Check sheet for the modelled part. Datum: model origin and axes. Units: mm. Coordinates: 2 decimals unless noted, no trailing zeros. Loops run counter-clockwise (first coordinate to the right, second up) from the corner with the lowest first, then second, coordinate; pieces in that order, holes last. Notation, with made-up numbers: M 87,-38.75 L 125,-38.75 A31 ccw 125,-1.75 Z; hole C 85.5,8 d3. An arc over 180 degrees is marked long. Return JSON: item names as keys, results as strings.
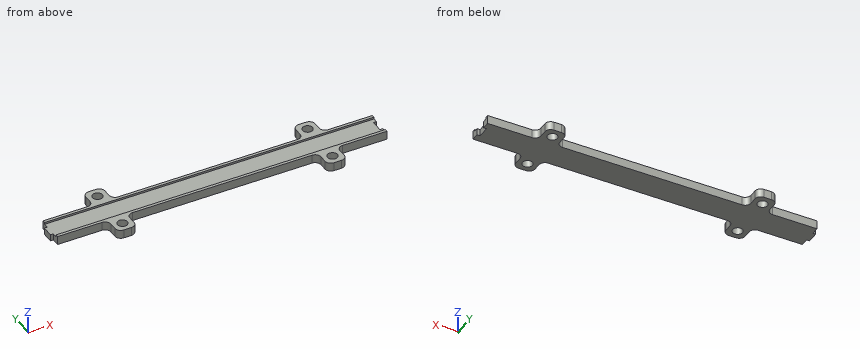
Autodesk Inventor part; units mm, degrees
ref_plane "YZ Plane" through (0, 0, 0) normal (1, 0, 0) x (0, 1, 0)
ref_plane "XZ Plane" through (0, 0, 0) normal (0, 1, 0) x (-1, 0, 0)
ref_plane "XY Plane" through (0, 0, 0) normal (0, 0, 1) x (1, 0, 0)
sketch "Skizze2" plane through (0, 0, 0) normal (0, 0, 1) x (1, 0, 0)
  line L0 (-86.25, 7) -> (86.25, 7)
  line L1 (86.25, 7) -> (86.25, -7)
  line L2 (86.25, -7) -> (-86.25, -7)
  line L3 (-86.25, -7) -> (-86.25, 7)
  line L4 (0, 9.8) -> (0, -9.8)
  line L5 (-120.75, 0) -> (120.75, 0)
  point P0 (0, 0)
  point P1 (-86.25, 0)
  point P2 (0, 7)
  dimension "d0" = 14
  dimension "d1" = 172.5
extrude "Extrusion1" add sketch "Skizze2" along normal blind 3.5
sketch "Skizze3" plane through (0, 0, 3.5) normal (0, 0, 1) x (1, 0, 0)
  line L0 (86.25, -7) -> (86.25, 7)
  line L1 (86.25, 7) -> (-86.25, 7)
  line L2 (-86.25, 7) -> (-86.25, -7)
  line L3 (-86.25, -7) -> (86.25, -7)
  line L4 (86.25, 7) -> (-86.25, 7)
  line L5 (-86.25, 7) -> (-86.25, 5.5)
  line L6 (-86.25, 5.5) -> (86.25, 5.5)
  line L7 (86.25, 5.5) -> (86.25, 7)
  line L8 (-86.25, 7) -> (-86.25, -7)
  line L9 (-86.25, -7) -> (86.25, -7)
  line L10 (86.25, -7) -> (86.25, -5.5)
  line L11 (86.25, -5.5) -> (-86.25, -5.5)
  line L12 (-86.25, -5.5) -> (-86.25, -7)
  point P0 (0, 0)
  dimension "d4" = 1.5
  dimension "d5" = 1.5
extrude "Extrusion2" add sketch "Skizze3" along normal blind 1 contours L3 L2 L11 L0 | L6 L2 L1 L0
sketch "Skizze4" plane through (0, 0, 0) normal (0, 0, -1) x (-1, 0, 0)
  line L0 (86.25, -7) -> (-86.25, -7)
  line L1 (155.9309, -7) -> (147.0048, -7)
  line L2 (60, -7) -> (50, -7)
  line L3 (50, -7) -> (50, -17)
  line L4 (50, -17) -> (60, -17)
  line L5 (60, -17) -> (60, -7)
  line L6 (50, 7) -> (60, 7)
  line L7 (60, 7) -> (60, 17)
  line L8 (60, 17) -> (50, 17)
  line L9 (50, 17) -> (50, 7)
  line L10 (86.25, -7) -> (-86.25, -7)
  line L11 (-86.25, 7) -> (86.25, 7)
  line L12 (86.25, 7) -> (86.25, -7)
  line L13 (-60, -9.0118) -> (-60, -17) construction
  line L14 (-60, -17) -> (-50, -17) construction
  line L15 (-50, -17) -> (-50, -7) construction
  line L16 (-86.25, -7) -> (-86.25, 7)
  point P0 (0, 0)
  point P1 (50, -7)
  point P2 (55, -17)
  point P3 (-55, -17)
  point P4 (55, -12)
  point P5 (55, 12)
  point P6 (60, -12)
  point P7 (60, 12)
  dimension "d8" = 10
  dimension "d9" = 10
  dimension "d30" = 110
  dimension "d31" = 10
  dimension "d32" = 24
  dimension "d33" = 55
extrude "Extrusion3" add sketch "Skizze4" against normal up to surface (4.5 mm away) contours L5 L4 L3 L0 | L6 L9 L8 L7
sketch "Skizze5" plane through (0, 0, 0) normal (0, 0, -1) x (-1, 0, 0)
  line L0 (50, -17) -> (60, -17)
  line L1 (50, -7) -> (50, -17)
  line L2 (50, 17) -> (50, 7)
  point P0 (0, 0)
  point P1 (55, -12)
  point P2 (55, 12)
  point P3 (55, -17)
  point P4 (50, -12)
  point P5 (50, 12)
  dimension "d13" = 24
hole "Bohrung1" at (-55, -12, 0) direction (0, 0, 1) diameter 5.2 end through all
fillet "Rundung1" radius 3 8 edges at (-60, -17, 2.25) (-50, -17, 2.25) (-50, -7, 2.25) (-60, -7, 2.25) (-50, 17, 2.25) (-60, 17, 2.25) (-50, 7, 2.25) (-60, 7, 2.25)
pattern_linear "Rechteckige Anordnung1" count 2 spacing 24 along (0, 1, 0) of "Bohrung1"
pattern_linear "Rechteckige Anordnung2" count 2 spacing 110 along (1, 0, 0) of "Rundung1", "Bohrung1", "Extrusion3", "Rechteckige Anordnung1"
sketch "Skizze7" plane through (0, 0, 3.5) normal (0, 0, 1) x (1, 0, 0)
  line L0 (-86.25, 5.5) -> (-86.25, -5.5)
  line L1 (-86.25, 3) -> (-87.75, 3)
  line L2 (-87.75, 3) -> (-87.75, -3)
  line L3 (-87.75, -3) -> (-86.25, -3)
  line L4 (-86.25, -3) -> (-86.25, 3)
  line L5 (86.25, -3.1) -> (84.65, -3.1)
  line L6 (84.65, -3.1) -> (84.65, 3.1)
  line L7 (84.65, 3.1) -> (86.25, 3.1)
  line L8 (86.25, 3.1) -> (86.25, -3.1)
  line L9 (86.25, -5.5) -> (86.25, 5.5)
  point P0 (0, 0)
  point P1 (-87.75, 0)
  point P2 (-86.25, 0)
  point P3 (-86.25, 0)
  point P4 (84.65, 0)
  point P5 (86.25, 0)
  point P6 (86.25, 0)
  dimension "d37" = 1.5
  dimension "d38" = 6
  dimension "d41" = 1.6
  dimension "d44" = 6.2
extrude "Extrusion5" add sketch "Skizze7" against normal up to surface (3.5 mm away) contours L0 L3 L2 L1
extrude "Extrusion6" cut sketch "Skizze7" against normal through all contours L5 L6 L7 L8
equation "\"d5\" = d4"
equation "\"d9\" = d8"
equation "\"d24\" = d13"
properties part number "LED_Strip_Halter" material "PA 6 schwarz"
1) Section check C-C on z = 2. Count the separate pieces of the cut face and the enclosed holes in it, then the cut area to 3 significant figures.
Answers:
{"separate pieces": "1", "enclosed holes": "4", "area": "2,730 mm²"}
2) Section check A-A on y = -12. Record the cut outline in (x, z).
Answers:
{"outline": "M -60,0 L -57.6,0 L -57.6,4.5 L -60,4.5 Z; M -52.4,0 L -50,0 L -50,4.5 L -52.4,4.5 Z; M 50,0 L 52.4,0 L 52.4,4.5 L 50,4.5 Z; M 57.6,0 L 60,0 L 60,4.5 L 57.6,4.5 Z"}
3) Section check B-B on x = -55. Record the cut outline in (y, z).
Answers:
{"outline": "M -17,0 L -14.6,0 L -14.6,4.5 L -17,4.5 Z; M -9.4,0 L 9.4,0 L 9.4,4.5 L 5.5,4.5 L 5.5,3.5 L -5.5,3.5 L -5.5,4.5 L -9.4,4.5 Z; M 14.6,0 L 17,0 L 17,4.5 L 14.6,4.5 Z"}
4) Section check D-D on x = 29. Record the cut outline in (y, z), then the cut area to 3 significant figures.
Answers:
{"outline": "M -7,0 L 7,0 L 7,4.5 L 5.5,4.5 L 5.5,3.5 L -5.5,3.5 L -5.5,4.5 L -7,4.5 Z", "area": "52.0 mm²"}
5) Scan lines: line 1 along X through (y, z) = (12, 3); line 2 along Y through (x, z) = (-55, 1.1); line 3 along X through (y, z) = (-13, 4.25). Record each from-to range of solid material in increasing order. Write a range as [from, to].
Answers:
{"line 1": "[-60, -57.6], [-52.4, -50], [50, 52.4], [57.6, 60]", "line 2": "[-17, -14.6], [-9.4, 9.4], [14.6, 17]", "line 3": "[-60, -57.4], [-52.6, -50], [50, 52.6], [57.4, 60]"}
6) Go/stop test with flat-tipped pins: pin 1 Ø1 at (y, z) = (-9, 3.5) entering from -X; pin 2 Ø2 at (x, z) = (-46, 1.5) entering from +Y; pin 3 Ø0.8 at (x, z) = (-37, 4) entering from -Y; pin 4 Ø4.5 at (x, y) = (-55, -12) entering from -Z. Record where each tip stops, or that it passes through.
Answers:
{"pin 1": "x = -60.4", "pin 2": "y = 7", "pin 3": "y = -7", "pin 4": "through"}
